```python
from build123d import *

# Parameters (mm, degrees)
SKETCH_1_W          = 20
SKETCH_1_H          = 20
EXTRUDE_1_DEPTH     = 20
SKETCH_2_R          = 3
CUT_EXTRUDE_1_DEPTH = 20
CUT_EXTRUDE_2_REACH = 32
SKETCH_3_R          = 3
CUT_EXTRUDE_3_REACH = 32
SKETCH_4_R          = 3
SKETCH_5_R          = 6
CUT_EXTRUDE_4_DEPTH = 18
SKETCH_6_R          = 6
CUT_EXTRUDE_5_DEPTH = 18
SKETCH_7_R          = 6
CUT_EXTRUDE_6_DEPTH = 18
CHAMFER_1_SIZE      = 1
CHAMFER_2_SIZE      = 1


with BuildPart() as part:
    # 草图1 → 凸台-拉伸1 (new body)
    with BuildSketch(Plane.XY):
        Rectangle(SKETCH_1_W, SKETCH_1_H)
    extrude(amount=EXTRUDE_1_DEPTH)

    # 草图2 → 切除-拉伸1 (cut)
    with BuildSketch(Plane(origin=(0, 0, 0), x_dir=(-1, 0, 0), z_dir=(0, 0, -1))):
        Circle(SKETCH_2_R)
    extrude(amount=-CUT_EXTRUDE_1_DEPTH, mode=Mode.SUBTRACT)

    # 切除-拉伸2: up to this face of the body (flat: up to its plane)
    cut_extrude_2_end = Plane(part.part.faces().sort_by_distance((-10, 0, 10))[0])
    # 草图3 → 切除-拉伸2 (cut, up to the picked face)
    with BuildSketch(Plane(origin=(10, 0, 0), x_dir=(0, 0, -1), z_dir=(1, 0, 0)), mode=Mode.PRIVATE) as cut_extrude_2_sk1:
        with Locations((-10, 0)):
            Circle(SKETCH_3_R)
    cut_extrude_2_tool1 = split(extrude(cut_extrude_2_sk1.sketch, amount=-CUT_EXTRUDE_2_REACH, mode=Mode.PRIVATE), bisect_by=cut_extrude_2_end, keep=Keep.BOTH, mode=Mode.PRIVATE)
    add(cut_extrude_2_tool1.solids().sort_by(Axis((10, 0, 10), (-1, 0, 0)))[0], mode=Mode.SUBTRACT)

    # 切除-拉伸3: up to this face of the body (flat: up to its plane)
    cut_extrude_3_end = Plane(part.part.faces().sort_by_distance((0, -10, 10))[0])
    # 草图4 → 切除-拉伸3 (cut, up to the picked face)
    with BuildSketch(Plane(origin=(0, 10, 0), x_dir=(1, 0, 0), z_dir=(0, 1, 0)), mode=Mode.PRIVATE) as cut_extrude_3_sk1:
        with Locations(Location((0, -10, 0), (0, 0, 270))):
            Circle(SKETCH_4_R)
    cut_extrude_3_tool1 = split(extrude(cut_extrude_3_sk1.sketch, amount=-CUT_EXTRUDE_3_REACH, mode=Mode.PRIVATE), bisect_by=cut_extrude_3_end, keep=Keep.BOTH, mode=Mode.PRIVATE)
    add(cut_extrude_3_tool1.solids().sort_by(Axis((0, 10, 10), (0, -1, 0)))[0], mode=Mode.SUBTRACT)

    # 草图5 → 切除-拉伸4 (cut)
    with BuildSketch(Plane(origin=(10, 0, 0), x_dir=(0, 0, -1), z_dir=(1, 0, 0))):
        with Locations((-10, 0)):
            Circle(SKETCH_5_R)
    extrude(amount=-CUT_EXTRUDE_4_DEPTH, mode=Mode.SUBTRACT)

    # 草图6 → 切除-拉伸5 (cut)
    with BuildSketch(Plane.XY.offset(20)):
        Circle(SKETCH_6_R)
    extrude(amount=-CUT_EXTRUDE_5_DEPTH, mode=Mode.SUBTRACT)

    # 草图7 → 切除-拉伸6 (cut)
    with BuildSketch(Plane.XZ.offset(10)):
        with Locations(Location((0, 10, 0), (0, 0, 270))):
            Circle(SKETCH_7_R)
    extrude(amount=-CUT_EXTRUDE_6_DEPTH, mode=Mode.SUBTRACT)

    # 倒角1
    chamfer_1_edges = [part.edges().sort_by_distance(p)[0] for p in [
        (0, -10, 20),
        (10, 0, 20),
        (10, -10, 10),
    ]]
    chamfer(chamfer_1_edges, length=CHAMFER_1_SIZE)

    # 倒角2
    chamfer_2_edges = [part.edges().sort_by_distance(p)[0] for p in [
        (10, 0, 16),
        (-6, 0, 20),
        (0, -10, 16),
    ]]
    chamfer(chamfer_2_edges, length=CHAMFER_2_SIZE)


solid = part.part
```
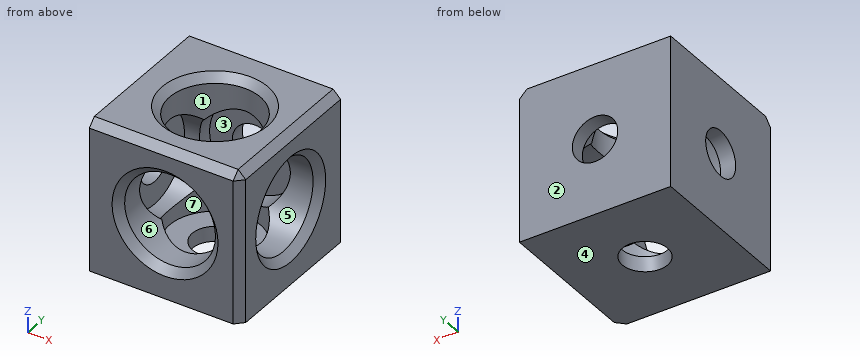
Input: part model. Units: mm. Frame: model coordinates. Face numbers are marked on the shaded views. A direction names the side the tool comes from. Give positions to 0.01 mm unless a question says otherwise; leave off trailing zeros. Write each loop counter-clockwise with the first axis right and the second up, starting at its lowest first coordinate (ties: lowest second). Pieces come first, ordered by that corner, then holes. Notation, with made-up numbers: (-7, 39.25) - (18, 39.25) arc R28 ccw to (18, 67.25) - close; hole circle Ø7 at (-19, 70). An arc over 180 degrees is marked (long way). Write item = value, one per line. Start each with the question number.
1. Section query A-A, the plane y = 0. Count the separate pieces of the cut face and the enclosed holes in it, then the cut area to 3 significant figures.
2. Section query D-D, the plane y = -8.5. Output: boundary loops of the cut face in (x, z), then the cut area to 3 significant figures.
3. Ray query, L1, parallel to X at y = -7.95, z = 10; L2, parallel to Y at x = -9.6, z = 10; L3, parallel to X at y = -4.5, z = 11. Return the intervals inside material, ascending.
4. Section query C-C, the plane z = 17.5. Output: boundary loops of the cut face in (x, y), then the cut area to 3 significant figures.
5. First-contact query: pin 1 Ø11 at (x, z) = (0, 10) entering from -Y; pin 2 Ø7 at (y, z) = (0, 10) entering from +X. Flat tips, straight axial feed; report the tip coordinate or a pass-through.
6. Mould query, pull axis Y, two halves, no side actions, for the marked faces 1, 2, 3 and 4. Classes: released by +Y, released by -Y, zero draft, split by the parting line, or undercut.
7. Access query for the marked faces 5, 6 and 7. Directions: +Z, -Z, +X, -X, +Y, -Y. A direction counts if a zero-diameter tool reaches every point of the face in a straight line with its end or side. Return the directions, or none.
Check sheet entries:
q1.separate_pieces = 4
q1.enclosed_holes = 0
q1.area = 85.5 mm2
q2.outline = (-10, 0) - (10, 0) - (10, 19) - (9, 20) - (-10, 20) - close; hole circle Ø12 at (0, 10)
q2.area = 286 mm2
q3.L1 = -10 to -6, 6 to 10
q3.L2 = -10 to -3, 3 to 10
q3.L3 = -10 to -8
q4.outline = (-10, -10) - (9, -10) - (10, -9) - (10, 10) - (-10, 10) - close; hole circle Ø12 at (0, 0)
q4.area = 286 mm2
q5.pin_1 = 8
q5.pin_2 = -8
q6.face_1 = undercut
q6.face_2 = released by +Y
q6.face_3 = released by -Y
q6.face_4 = zero draft
q7.face_5 = +X
q7.face_6 = -Y
q7.face_7 = +Z
